The listing builds one solid part. Answer for the finished solid, in the listing's coordinates (mm). Face numbers are marked on the shaded views. Coordinates: 2 decimals unless noted, no trailing zeros. Loops run counter-clockwise (first coordinate to the right, second up) from the corner with the lowest first, then second, coordinate; pieces in that order, holes last. Notation, with made-up numbers: (-40, -0.5) - (-25, -0.5) arc R15 ccw to (-25, 10.5) - close; hole circle Ø7 at (-31, -18.75). An arc over 180 degrees is marked (long way). Put each result on its own line as item: value.
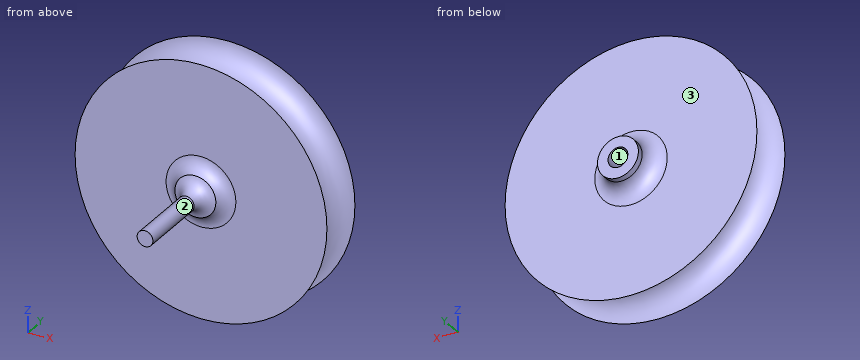
Autodesk Inventor part; units mm, degrees
ref_plane "YZ Plane" through (0, 0, 0) normal (1, 0, 0) x (0, 1, 0)
ref_plane "XZ Plane" through (0, 0, 0) normal (0, 1, 0) x (-1, 0, 0)
ref_plane "XY Plane" through (0, 0, 0) normal (0, 0, 1) x (1, 0, 0)
sketch "Sketch1" plane through (0, 0, 0) normal (0, 1, 0) x (-1, 0, 0)
  circle A0 centre (0, 0) radius 40
  dimension "d0" = 80
extrude "Extrusion1" add sketch "Sketch1" along normal blind 15
sketch "Sketch2" plane through (0, 0, 0) normal (1, 0, 0) x (0, 1, 0)
  line L0 (0, 40) -> (15, 40)
  line L1 (15, -40) -> (15, 40)
  circle A0 centre (7.5, 40) radius 7.5
  point P0 (0, 0)
sketch3d "3D Sketch1"
  arc A0 (-40, 15, 0) -> (0, 15, 40) centre (0, 15, 0) ccw
  arc A1 (0, 15, 40) -> (40, 15, 0) centre (0, 15, 0) ccw
  arc A2 (40, 15, 0) -> (0, 15, -40) centre (0, 15, 0) ccw
  arc A3 (0, 15, -40) -> (-40, 15, 0) centre (0, 15, 0) ccw
sweep "Sweep1" cut profiles "Sketch2" path "3D Sketch1" picked at (7.8013, 37.5182) contours L0 A0
sketch "Sketch3" plane through (0, 15, 0) normal (0, 1, 0) x (1, 0, 0)
  circle A0 centre (0, 0) radius 3.15
  circle A1 centre (0, 0) radius 6.5
  dimension "d5" = 6.3
  dimension "d6" = 13
extrude "Extrusion2" add sketch "Sketch3" along normal blind 7
sketch "Sketch4" plane through (0, 0, 0) normal (0, -1, 0) x (1, 0, 0)
  circle A0 centre (0, 0) radius 3.15
  circle A1 centre (0, 0) radius 6.5
  dimension "d9" = 13
extrude "Extrusion3" add sketch "Sketch4" along normal blind 3 contours A0 | A1
sketch "Sketch5" plane through (0, 15, 0) normal (0, 1, 0) x (1, 0, 0)
  circle A0 centre (0, 0) radius 3.15
  circle A1 centre (0, 0) radius 3.15
  dimension "d12" = 6.3
extrude "Extrusion4" cut sketch "Sketch5" against normal blind 15
sketch "Sketch6" plane through (0, -3, 0) normal (0, -1, 0) x (1, 0, 0)
  circle A0 centre (0, 0) radius 3.15
  circle A1 centre (0, 0) radius 2.5
  dimension "d15" = 5
extrude "Extrusion5" add sketch "Sketch6" along normal blind 27 contours A1
fillet "Fillet1" radius 5 1 edges at (-2.5, -3, 0)
fillet "Fillet2" radius 5 1 edges at (-6.5, 0, 0)
fillet "Fillet3" radius 5 1 edges at (-6.5, 15, 0)
properties part number "pulley"
1) The part is cut by section D-D (y = -4). Give the vertices of the cut face in (x, z).
Found:
outline: circle Ø8.74 at (0, 0)
2) The part is cut by section C-C (y = -13.5). Give the vertices of the cut face in (x, z).
Found:
outline: circle Ø5 at (0, 0)
3) The part is cut by section B-B (x = 0). Give the vertices of the cut face in (y, z), and give its area (3 significant figures).
Found:
outline: (-30, -2.5) - (-7.9, -2.5) arc R5 cw to (-3, -6.5) arc R5 cw to (0, -11.08) - (0, -40) arc R7.5 cw to (15, -40) - (15, -11.5) arc R5 cw to (20, -6.5) - (22, -6.5) - (22, -3.15) - (0, -3.15) - (0, 3.15) - (22, 3.15) - (22, 6.5) - (20, 6.5) arc R5 cw to (15, 11.5) - (15, 40) arc R7.5 cw to (0, 40) - (0, 11.08) arc R5 cw to (-3, 6.5) arc R5 cw to (-7.9, 2.5) - (-30, 2.5) - close
area: 1,180 mm^2
4) For a pull along X with two mould halves and no side action, classify the marked faces 1, 2 and 3 as pulls with the +X half, pulls with the -X half, needs draft (parallel to the pull), parting line crosses it, or undercut.
Found:
face 1: undercut
face 2: parting line crosses it
face 3: needs draft
5) Each of these flat-tipped pins is pushed along its axis until it touches: pin 1 (6 mm diameter, centred on x = -19.5, z = 7.5, fed in from +Y); pin 2 (5 mm diameter, centred on x = -24.5, y = 10.5, fed in from +Z); pin 3 (1 mm diameter, centred on x = -11, y = 13.5, fed in from -Z); pin 4 (8 mm diameter, centred on x = -8.5, y = -15.5, fed in from -Z). Where does it stop, or does it pass through?
Found:
pin 1: stops at y = 15
pin 2: stops at z = 25.59
pin 3: stops at z = -34.56
pin 4: passes through
6) The part is cut by section A-A (z = 0). Give the vertices of the cut face in (x, y).
Found:
outline: (-40, 0) - (-11.08, 0) arc R5 cw to (-6.5, -3) arc R5 cw to (-2.5, -7.9) - (-2.5, -30) - (2.5, -30) - (2.5, -7.9) arc R5 cw to (6.5, -3) arc R5 cw to (11.08, 0) - (40, 0) arc R7.5 cw to (40, 15) - (11.5, 15) arc R5 cw to (6.5, 20) - (6.5, 22) - (3.15, 22) - (3.15, 0) - (-3.15, 0) - (-3.15, 22) - (-6.5, 22) - (-6.5, 20) arc R5 cw to (-11.5, 15) - (-40, 15) arc R7.5 cw to start
7) Straight lines are drawn through the part: L1, parallel to Y at x = 15.5, z = 27; L2, parallel to Y at x = 31, z = -17.5; L3, parallel to Z at x = -0.5, y = 18. For each, find the intervals that lie inside material, in ascending order. Write a range as [from, to].
Found:
L1: y = [0, 15]
L2: y = [0, 1.43], [13.57, 15]
L3: z = [-6.9, -3.11], [3.11, 6.9]
